Work out the finished part from the listing and answer in its coordinate system (mm). Round coordinates to 2 decimals unless told otherwise and drop trailing zeros. Write each loop counter-clockwise with the first axis right and the second up, starting at its lowest first coordinate (ties: lowest second). Pieces come first, ordered by that corner, then holes. Notation, with made-up numbers: M 9,41 L 21,41 A13 ccw 21,58 Z; hole C -23.5,25 d1. An arc over 180 degrees is marked long. One line per item, written item: value. Start each with the question number.
Q1. Find section C-C (x = 8). Write down the section's boundary in (y, z).
Q2. Given pin 1 Ø1.5 at (y, z) = (2, -215.5) entering from +X; pin 2 Ø2.5 at (y, z) = (3, -123.5) entering from -X; pin 3 Ø1.5 at (x, y) = (85.5, 1) entering from +Z; pin 4 Ø2.5 at (x, z) = (234.5, -135) entering from +Y, each flat-ended and moving along its own axis, determine where each tip first touches the part or whether it passes through.
Q3. Find section A-A (z = -237). Write down the section's boundary in (x, y), and give its area (4 significant figures).
Q4. Find section B-B (z = -8). Write down the section's boundary in (x, y).
Q5. Consider probe 1 along X at (y, z) = (1.9, -8); probe 2 along Z at (x, y) = (15.5, 1.9); probe 3 along Z at (x, y) = (235, 2.05). Determine where each line is inside the solid, lowest interval first.
Q6. Find section D-D (y = 3). Count the separate pieces of the cut face and the enclosed holes in it, and give its area (3 significant figures).
Q7. The mould has two halves that part along Z. Classify faces 1 (the cylindrical face through (8.143, 2.535, -240.247)), 2 (the flat face through (152, 5, -124)): released by +Z, released by -Z, zero draft, split by the parting line, or undercut.
from build123d import *

# Parameters (mm, degrees)
SKETCH1_W                           = 250
SKETCH1_H                           = 250
SKETCH1_W_2                         = 4.8
SKETCH1_H_2                         = 20
SKETCH1_W_3                         = 10
SKETCH1_H_3                         = 2.9
SKETCH1_W_4                         = 2.9
SKETCH1_H_4                         = 30
SKETCH1_H_5                         = 50
SKETCH1_W_5                         = 6
SKETCH1_H_6                         = 70
BOSS_EXTRUDE1_DEPTH                 = 5
SKETCH2_R                           = 2.5
CUT_EXTRUDE1_DEPTH                  = 354.588744165
SKETCH3_R                           = 3.25
CUT_EXTRUDE2_DEPTH                  = 354.588744165
SKETCH4_W                           = 5
SKETCH4_H                           = 20
SKETCH4_W_2                         = 20
SKETCH4_H_2                         = 5
BOSS_EXTRUDE2_DEPTH                 = 5
F_4_5_4_5_DIAMETER_HOLE1_AT_2_COUNT = 2
F_4_5_4_5_DIAMETER_HOLE1_AT_2_PITCH = 50
F_4_5_4_5_DIAMETER_HOLE1_AT_3_COUNT = 2
F_4_5_4_5_DIAMETER_HOLE1_AT_3_PITCH = 130
F_4_5_4_5_DIAMETER_HOLE1_AT_4_COUNT = 2
F_4_5_4_5_DIAMETER_HOLE1_AT_4_PITCH = 120
SKETCH9_W                           = 4.8
SKETCH9_H                           = 20
CUT_EXTRUDE3_DEPTH                  = 358.141428569
SKETCH10_R                          = 2.1
CUT_EXTRUDE4_DEPTH                  = 5


with BuildPart() as part:
    # Sketch1 → Boss-Extrude1 (new body)
    with BuildSketch(Plane(origin=(0, 0, 0), x_dir=(1, 0, 0), z_dir=(0, 1, 0))):
        with Locations((125, 125)):
            Rectangle(SKETCH1_W, SKETCH1_H)
        with Locations((142.5, 15)):
            Rectangle(SKETCH1_W_2, SKETCH1_H_2, mode=Mode.SUBTRACT)
        with Locations((107.5, 15)):
            Rectangle(SKETCH1_W_2, SKETCH1_H_2, mode=Mode.SUBTRACT)
        with Locations((92, 53.93422616)):
            Rectangle(SKETCH1_W_3, SKETCH1_H_3, mode=Mode.SUBTRACT)
        with Locations((103.55, 79.434226159)):
            Rectangle(SKETCH1_W_4, SKETCH1_H_4, mode=Mode.SUBTRACT)
        with Locations((92, 104.93422616)):
            Rectangle(SKETCH1_W_3, SKETCH1_H_3, mode=Mode.SUBTRACT)
        with Locations((107.5, 125)):
            Rectangle(SKETCH1_W_2, SKETCH1_H_2, mode=Mode.SUBTRACT)
        with Locations((142.5, 125)):
            Rectangle(SKETCH1_W_2, SKETCH1_H_2, mode=Mode.SUBTRACT)
        with Locations((225, 200)):
            Rectangle(SKETCH1_W_2, SKETCH1_H_5, mode=Mode.SUBTRACT)
        with Locations((125, 135)):
            Rectangle(SKETCH1_W_5, SKETCH1_H_6, mode=Mode.SUBTRACT)
        with Locations((25, 200)):
            Rectangle(SKETCH1_W_2, SKETCH1_H_5, mode=Mode.SUBTRACT)
    extrude(amount=BOSS_EXTRUDE1_DEPTH)

    # Sketch2 → Cut-Extrude1 (cut, through all)
    with BuildSketch(Plane(origin=(0, 5, 0), x_dir=(1, 0, 0), z_dir=(0, 1, 0))):
        with Locations(Location((15, 100, 0), (0, 0, 270))):
            Circle(SKETCH2_R)
        with Locations(Location((63, 100, 0), (0, 0, 270))):
            Circle(SKETCH2_R)
    cut_extrude1 = extrude(amount=-CUT_EXTRUDE1_DEPTH, mode=Mode.SUBTRACT)

    # Sketch3 → Cut-Extrude2 (cut, through all)
    with BuildSketch(Plane(origin=(0, 5, 0), x_dir=(1, 0, 0), z_dir=(0, 1, 0))):
        with Locations(Location((8, 8, 0), (0, 0, 270))):
            Circle(SKETCH3_R)
        with Locations(Location((8, 237, 0), (0, 0, 270))):
            Circle(SKETCH3_R)
    cut_extrude2 = extrude(amount=-CUT_EXTRUDE2_DEPTH, mode=Mode.SUBTRACT)

    # Mirror1: Cut-Extrude2 across plane
    add(cut_extrude2.mirror(Plane.ZY.offset(-125)), mode=Mode.SUBTRACT)

    # Sketch4 → Boss-Extrude2 (add)
    with BuildSketch(Plane(origin=(0, 5, 0), x_dir=(1, 0, 0), z_dir=(0, 1, 0))):
        with Locations((-2.5, 190)):
            Rectangle(SKETCH4_W, SKETCH4_H)
        with Locations((-2.5, 60)):
            Rectangle(SKETCH4_W, SKETCH4_H)
        with Locations((60, -2.5)):
            Rectangle(SKETCH4_W_2, SKETCH4_H_2)
    boss_extrude2 = extrude(amount=-BOSS_EXTRUDE2_DEPTH)

    # Mirror2: Boss-Extrude2 across plane
    add(boss_extrude2.mirror(Plane.ZY.offset(-125)))

    # Mirror3: Cut-Extrude1 across plane
    add(cut_extrude1.mirror(Plane.ZY.offset(-125)), mode=Mode.SUBTRACT)

    # Sketch6 → Ø4.5 (4.5) Diameter Hole1 (revolve, cut)
    with BuildSketch(Plane(origin=(15.5, 5, -135), x_dir=(0, 0, 1), z_dir=(1, 0, 0))):
        Polygon((0, 0), (0, 11.351936393), (2.25, 10), (2.25, 0), align=None)
    f_4_5_4_5_diameter_hole1 = revolve(axis=Axis((15.5, 11.35, -135), (0, -1, 0)), mode=Mode.SUBTRACT)

    # Ø4.5 (4.5) Diameter Hole1 at 2: Ø4.5 (4.5) Diameter Hole1 ×2
    with Locations(*[(i * F_4_5_4_5_DIAMETER_HOLE1_AT_2_PITCH, 0, 0) for i in range(1, F_4_5_4_5_DIAMETER_HOLE1_AT_2_COUNT)]):
        add(f_4_5_4_5_diameter_hole1, mode=Mode.SUBTRACT)

    # Ø4.5 (4.5) Diameter Hole1 at 3: Ø4.5 (4.5) Diameter Hole1 ×2
    with Locations(*[Vector(0.38461538461538475, 0, 0.9230769230769231) * (i * F_4_5_4_5_DIAMETER_HOLE1_AT_3_PITCH) for i in range(1, F_4_5_4_5_DIAMETER_HOLE1_AT_3_COUNT)]):
        add(f_4_5_4_5_diameter_hole1, mode=Mode.SUBTRACT)

    # Ø4.5 (4.5) Diameter Hole1 at 4: Ø4.5 (4.5) Diameter Hole1 ×2
    with Locations(*[(0, 0, i * F_4_5_4_5_DIAMETER_HOLE1_AT_4_PITCH) for i in range(1, F_4_5_4_5_DIAMETER_HOLE1_AT_4_COUNT)]):
        add(f_4_5_4_5_diameter_hole1, mode=Mode.SUBTRACT)

    # Mirror4: Ø4.5 (4.5) Diameter Hole1 across plane
    add(f_4_5_4_5_diameter_hole1.mirror(Plane.ZY.offset(-125)), mode=Mode.SUBTRACT)

    # Mirror4 copy 1 sketch → Mirror4 copy 1 (revolve, cut)
    with BuildSketch(Plane(origin=(184.5, 5, -135), x_dir=(0, 0, 1), z_dir=(-1, 0, 0))):
        Polygon((0, 0), (0, -11.351936393), (2.25, -10), (2.25, 0), align=None)
    revolve(axis=Axis((184.5, 11.35, -135), (0, 1, 0)), mode=Mode.SUBTRACT)

    # Mirror4 copy 2 sketch → Mirror4 copy 2 (revolve, cut)
    with BuildSketch(Plane(origin=(184.5, 5, -15), x_dir=(0, 0, 1), z_dir=(-1, 0, 0))):
        Polygon((0, 0), (0, -11.351936393), (2.25, -10), (2.25, 0), align=None)
    revolve(axis=Axis((184.5, 11.35, -15), (0, 1, 0)), mode=Mode.SUBTRACT)

    # Mirror4 copy 3 sketch → Mirror4 copy 3 (revolve, cut)
    with BuildSketch(Plane(origin=(234.5, 5, -15), x_dir=(0, 0, 1), z_dir=(-1, 0, 0))):
        Polygon((0, 0), (0, -11.351936393), (2.25, -10), (2.25, 0), align=None)
    revolve(axis=Axis((234.5, 11.35, -15), (0, 1, 0)), mode=Mode.SUBTRACT)

    # Sketch9 → Cut-Extrude3 (cut, through all)
    with BuildSketch(Plane.XZ):
        with Locations((107.5, -185)):
            Rectangle(SKETCH9_W, SKETCH9_H)
    cut_extrude3 = extrude(amount=-CUT_EXTRUDE3_DEPTH, mode=Mode.SUBTRACT)

    # Mirror5: Cut-Extrude3 across plane
    add(cut_extrude3.mirror(Plane.ZY.offset(-125)), mode=Mode.SUBTRACT)

    # Sketch10 → Cut-Extrude4 (cut)
    with BuildSketch(Plane.XZ):
        with Locations(Location((15, -210, 0), (0, 0, 270))):
            Circle(SKETCH10_R)
        with Locations(Location((235, -210, 0), (0, 0, 270))):
            Circle(SKETCH10_R)
    extrude(amount=-CUT_EXTRUDE4_DEPTH, mode=Mode.SUBTRACT)


solid = part.part
The answers:
1. outline: M 0,-250 L 5,-250 L 5,-240.25 L 0,-240.25 Z; M 0,-233.75 L 5,-233.75 L 5,-11.25 L 0,-11.25 Z; M 0,-4.75 L 5,-4.75 L 5,0 L 0,0 Z
2. pin 1: x = 250
2. pin 2: x = 0
2. pin 3: z = 0
2. pin 4: through
3. outline: M 0,0 L 4.75,0 L 4.75,5 L 0,5 Z; M 11.25,0 L 238.75,0 L 238.75,5 L 11.25,5 Z; M 245.25,0 L 250,0 L 250,5 L 245.25,5 Z
3. area: 1,185 mm2
4. outline: M 0,0 L 4.75,0 L 4.75,5 L 0,5 Z; M 11.25,0 L 105.1,0 L 105.1,5 L 11.25,5 Z; M 109.9,0 L 140.1,0 L 140.1,5 L 109.9,5 Z; M 144.9,0 L 238.75,0 L 238.75,5 L 144.9,5 Z; M 245.25,0 L 250,0 L 250,5 L 245.25,5 Z
5. probe 1: 0 to 4.75, 11.25 to 105.1, 109.9 to 140.1, 144.9 to 238.75, 245.25 to 250
5. probe 2: -250 to -212.04, -207.96 to -137.25, -132.75 to -102.45, -97.55 to -17.25, -12.75 to 0
5. probe 3: -250 to -212.1, -207.9 to -137.19, -132.81 to -102.5, -97.5 to -17.19, -12.81 to 0
6. separate pieces: 1
6. enclosed holes: 30
6. area: 61,100 mm2
7. face 1: undercut
7. face 2: zero draft
